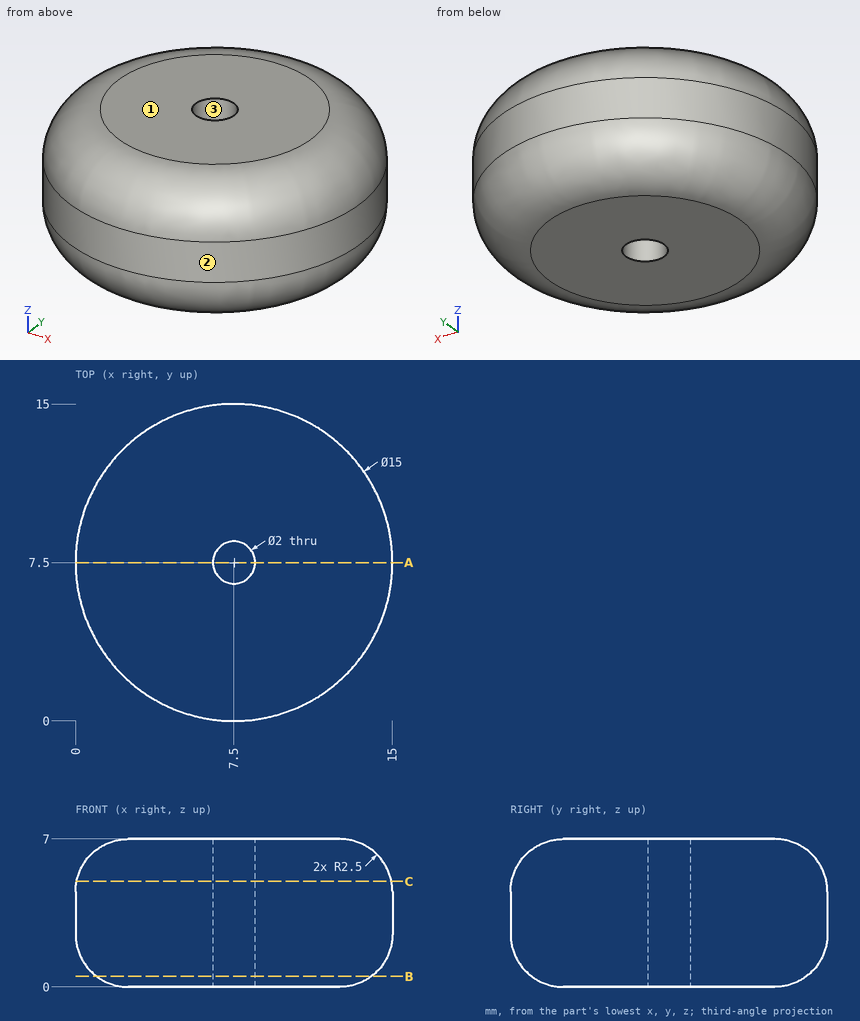
Can you work these out from the drawing? Everything is in mm from the part's minimum corner. Round coordinates to 2 decimals unless told otherwise and drop trailing zeros. Order: outer loops, then holes, each group sorted by start corner. A loop starts at its lowest first (then second) coordinate and runs counter-clockwise, first axis right, second up.
(1) I'm going to push flat-ended pins straight in: pin 1 (2 mm diameter, centred on x = 3, y = 12, fed in from -Z); pin 2 (4 mm diameter, centred on x = 3.5, z = 6, fed in from -Y); pin 3 (3 mm diameter, centred on y = 6, z = 1, fed in from -X); pin 4 (1.8 mm diameter, centred on x = 7.5, y = 7.5, fed in from +Z). Where does each tip first touch, or does it pass through?
Results are:
pin 1: stops at z = 0.03
pin 2: stops at y = 0.4
pin 3: stops at x = 0.04
pin 4: passes through
(2) We'd pull the mould along X, two halves only. Please class the marked faces 1, 2 and 3: +X half, -X half, draft (parallel to the pull), parting line (faces both ways), or undercut.
Results are:
face 1: draft
face 2: parting line
face 3: undercut
(3) If we section it at A-A (y = 7.5): Please give me the cut outline in (x, z), plus the area to 3 significant figures.
Results are:
outline: (0, 2.5) arc R2.5 ccw to (2.5, 0) - (6.5, 0) - (6.5, 7) - (2.5, 7) arc R2.5 ccw to (0, 4.5) - close; (8.5, 0) - (12.5, 0) arc R2.5 ccw to (15, 2.5) - (15, 4.5) arc R2.5 ccw to (12.5, 7) - (8.5, 7) - close
area: 85.6 mm2
(4) If we section it at B-B (z = 0.5): Please give me the cut outline in (x, y).
Results are:
outline: circle Ø13 at (7.5, 7.5); hole circle Ø2 at (7.5, 7.5)
(5) If I drill on L1, parallel to Y at x = 7.5, z = 4; L2, parallel to Y at x = 7.5, z = 5.75; L3, parallel to X at y = 8, z = 3.5, over which ranges is the centre line in solid material (lowest first)?
Results are:
L1: y = 0 to 6.5, 8.5 to 15
L2: y = 0.33 to 6.5, 8.5 to 14.67
L3: x = 0.02 to 6.63, 8.37 to 14.98
(6) If we section it at C-C (z = 5): Please give me the cut outline in (x, y).
Results are:
outline: circle Ø14.9 at (7.5, 7.5); hole circle Ø2 at (7.5, 7.5)
